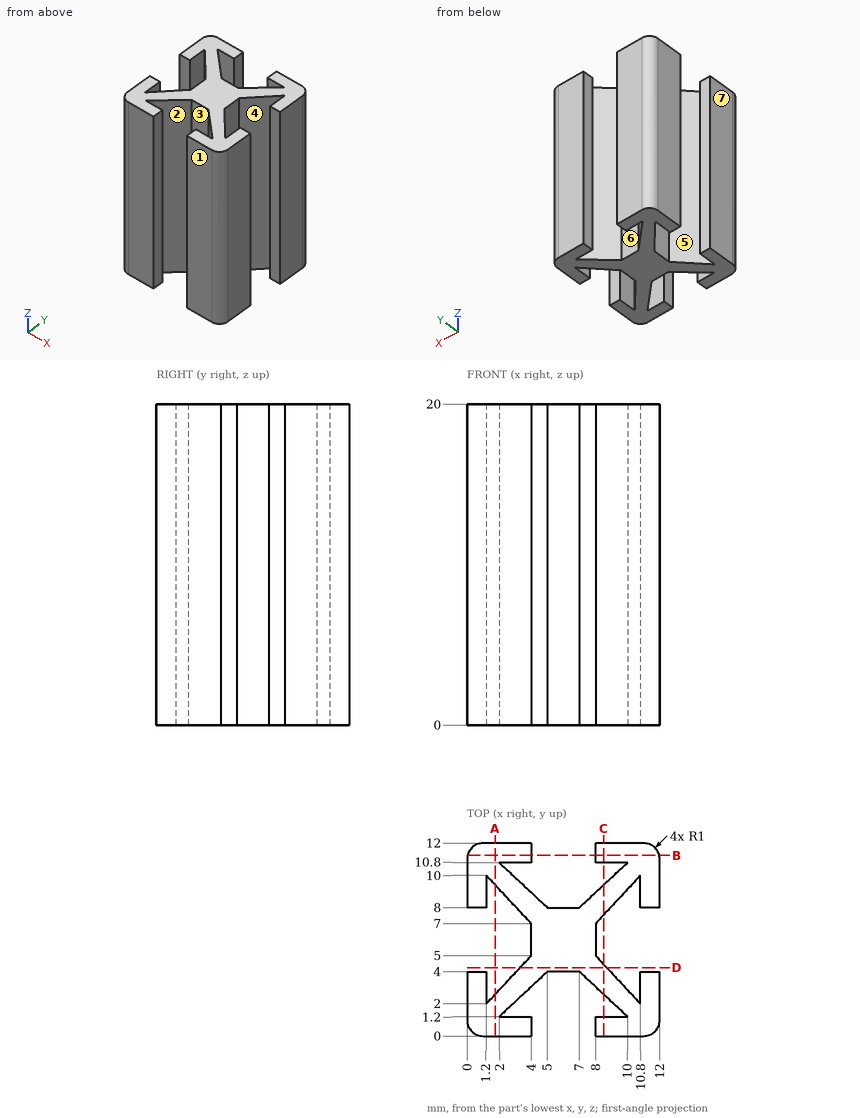
Geometry check sheet. Reference: drawing and pictorial views, mm from the part's lowest x, y, z. A direction names the side the tool comes from. Give positions to 0.01 mm unless a question says otherwise; leave off trailing zeros. Order: outer loops, then holes, each group sorted by start corner. A loop starts at its lowest first (then second) coordinate and runs counter-clockwise, first axis right, second up. Notation, with made-up numbers: M 76,87 L 104,87 A32 ccw 104,119 Z; hole C -24,-17.75 d3. An arc over 180 degrees is marked long. Answer as a JSON object with one key per item and string values. Group by question number.
1) Cross-section at A-A (x = 1.75). Enter the section's corners in (y, z).
2) Mould release check, pull along Y, two halves, no side actions. Record for the marked faces 4, 5, 6 and 7: released by +Y, released by -Y, zero draft, split by the parting line, or undercut.
3) Cross-section at D-D (y = 4.25). Enter the section's corners in (x, z).
4) Depth check by flat-ended pin: pin 1 Ø1 at (y, z) = (6, 14.5) entering from -X; pin 2 Ø0.6 at (y, z) = (0.5, 6.5) entering from +X; pin 3 Ø0.6 at (x, z) = (11.5, 10) entering from +Y. Enter the tip coordinate at first touch or a pass-through.
5) Cross-section at C-C (x = 8.5). Enter the section's corners in (y, z), then the cut area to 3 significant figures.
6) Access from +Z, -Z, +X, -X, +Y, -Y to the whole of each face (thin tool, end or side, straight path). Record for the marked faces 1, 2 and 3.
7) Cross-section at B-B (y = 11.25). Enter the section's corners in (x, z), then the cut area to 3 significant figures.
8) Scan lines: line 1 along Y through (x, z) = (2.25, 2) (3 decimals); line 2 along Y through (x, z) = (11, 9.75); line 3 along Y through (x, z) = (9.5, 14). Record each from-to range of solid material in increasing order. Write a range as [from, to].
Result sheet:
{
 "1": {"outline": "M 0,0 L 2.59,0 L 2.59,20 L 0,20 Z; M 9.41,0 L 12,0 L 12,20 L 9.41,20 Z"},
 "2": {"face 4": "undercut", "face 5": "undercut", "face 6": "released by +Y", "face 7": "zero draft"},
 "3": {"outline": "M 3.3,0 L 8.7,0 L 8.7,20 L 3.3,20 Z"},
 "4": {"pin 1": "stops at x = 4", "pin 2": "stops at x = 11.98", "pin 3": "stops at y = 11.98"},
 "5": {"outline": "M 0,0 L 1.2,0 L 1.2,20 L 0,20 Z; M 2.6,0 L 4.46,0 L 4.46,20 L 2.6,20 Z; M 7.54,0 L 9.4,0 L 9.4,20 L 7.54,20 Z; M 10.8,0 L 12,0 L 12,20 L 10.8,20 Z", "area": "123 mm2"},
 "6": {"face 1": "+Z, -Z, +X, -X, -Y", "face 2": "+Z, -Z", "face 3": "+Z, -Z, -Y"},
 "7": {"outline": "M 0.03,0 L 4,0 L 4,20 L 0.03,20 Z; M 8,0 L 11.97,0 L 11.97,20 L 8,20 Z", "area": "159 mm2"},
 "8": {"line 1": "y = [0, 1.2], [1.433, 3.125], [8.875, 10.567], [10.8, 12]", "line 2": "y = [0, 4], [8, 12]", "line 3": "y = [0, 1.2], [1.67, 3.39], [8.61, 10.33], [10.8, 12]"}
}
